from build123d import *

# Parameters (mm, degrees)
ESQUISSE4_R        = 4
ESQUISSE4_R_2      = 3
BOSS_EXTRU_1_DEPTH = 6
ESQUISSE6_R        = 3
ESQUISSE6_R_2      = 1.5
BOSS_EXTRU_2_DEPTH = 1
BOSS_EXTRU_3_DEPTH = 2


with BuildPart() as part:
    # Esquisse4 → Boss.-Extru.1 (new body)
    with BuildSketch(Plane.XY):
        Circle(ESQUISSE4_R)
        Circle(ESQUISSE4_R_2, mode=Mode.SUBTRACT)
    extrude(amount=BOSS_EXTRU_1_DEPTH)

    # Esquisse6 → Boss.-Extru.2 (add)
    with BuildSketch(Plane.XY.offset(6)):
        Circle(ESQUISSE6_R)
        Circle(ESQUISSE6_R_2, mode=Mode.SUBTRACT)
    extrude(amount=-BOSS_EXTRU_2_DEPTH)

    # Esquisse7 → Boss.-Extru.3 (add)
    with BuildSketch(Plane.XY.offset(6)):
        with BuildLine():
            ThreePointArc((3.464101615, 2), (3.863703305, 1.03527618), (4, 0))
            ThreePointArc((4, 0), (3.870082468, -1.011168479), (3.488769153, -1.956652702))
            Line((3.488769153, -1.956652702), (3.505079435, -2))
            Line((3.505079435, -2), (10.76772807, -2))
            Line((10.76772807, -2), (20.627571531, 6.877842929))
            ThreePointArc((20.627571531, 6.877842929), (20.775599969, 9.702393792), (17.951049106, 9.85042223))
            Line((17.951049106, 9.85042223), (9.23227193, 2))
            Line((9.23227193, 2), (3.464101615, 2))
        make_face()
        with BuildLine():
            ThreePointArc((0, 4), (1.03527618, 3.863703305), (2, 3.464101615))
            Line((2, 3.464101615), (2, 9.23227193))
            Line((2, 9.23227193), (9.85042223, 17.951049106))
            ThreePointArc((9.85042223, 17.951049106), (9.702393792, 20.775599969), (6.877842929, 20.627571531))
            Line((6.877842929, 20.627571531), (-2, 10.76772807))
            Line((-2, 10.76772807), (-2, 3.464101615))
            ThreePointArc((-2, 3.464101615), (-1.03527618, 3.863703305), (0, 4))
        make_face()
    extrude(amount=-BOSS_EXTRU_3_DEPTH)


solid = part.part
Input: part model. Units: mm. Frame: model coordinates. A direction names the side the tool comes from. Round coordinates to 2 decimals unless told otherwise and drop trailing zeros. Loops run counter-clockwise (first coordinate to the right, second up) from the corner with the lowest first, then second, coordinate; pieces in that order, holes last. Notation, with made-up numbers: (-31.5, 81) -> (10.5, 81) arc R22 cw to (10.5, 88) -> close; hole circle Ø2 at (50, 6.25). An arc over 180 degrees is marked (long way). Answer as a JSON object with one key per item and string values. Group by question number.
1) Pin query (flat end, axial travel): pin 1 (10 mm diameter, centred on x = 7.5, y = 7.5, fed in from +Z); pin 2 (1.6 mm diameter, centred on x = 6, z = 4.5, fed in from -Y); pin 3 (1.6 mm diameter, centred on y = 8.5, z = 5, fed in from -X); pin 4 (10 mm diameter, centred on x = 15.5, y = 3.5, fed in from -Z). Return the tip coordinate at first contact, or that it passes through.
2) Ray query, L1, parallel to Y at x = 0, z = 3.2; L2, parallel to Z at x = -1.5, y = -2.5; L3, parallel to Z at x = 19.75, y = 6.5. Return the intervals inside material, ascending.
3) Reachability of faces 5 (the cylindrical face through (-3, 0, 2)), 6 (the flat face through (10, 2, 6)), 7 (the flat face through (-2, 7, 5)), 8 (the flat face through (2, 6, 5)), 9 (the flat face through (7, -2, 5)) from +Z, -Z, +X, -X, +Y, -Y: full face, straight path, thin tool, end or side. Return the list, or none.
4) Section query A-A on z = 5.3. Output: boundary loops of the cut face in (x, y), plus the area to 3 significant figures.
5) Section query D-D on x = 8. Output: boundary loops of the cut face in (y, z).
6) Section query B-B on x = 0. Output: boundary loops of the cut face in (y, z).
7) Draft query along X for faces 1 (the flat face through (6, 2, 5)), 2 (the cylindrical face through (9.73, 20.75, 5.01)), 3 (the flat face through (1, 3, 0)), 4 (the flat face through (15.63, 2.38, 5.01)). Return one class per face: +X half, -X half, draft (parallel to the pull), parting line (faces both ways), or undercut.
Reply:
{
 "1": {"pin 1": "passes through", "pin 2": "stops at y = -2", "pin 3": "stops at x = -2", "pin 4": "stops at z = 4"},
 "2": {"L1": "y = -4 to -3, 3 to 4", "L2": "z = 5 to 6", "L3": "z = 4 to 6"},
 "3": {"face 5": "-Z", "face 6": "+Z, +X, -X, +Y, -Y", "face 7": "+Z, -Z, -X, +Y", "face 8": "+Z, -Z", "face 9": "+Z, -Z, +X, -Y"},
 "4": {"outline": "(-2, 3.46) arc R4 ccw (long way) to (3.49, -1.96) -> (3.51, -2) -> (10.77, -2) -> (20.63, 6.88) arc R2 ccw to (17.95, 9.85) -> (9.23, 2) -> (3.46, 2) arc R4 ccw to (2, 3.46) -> (2, 9.23) -> (9.85, 17.95) arc R2 ccw to (6.88, 20.63) -> (-2, 10.77) -> close; hole circle Ø3 at (0, 0)", "area": "205 mm2"},
 "5": {"outline": "(-2, 4) -> (2, 4) -> (2, 6) -> (-2, 6) -> close; (15.9, 4) -> (21.26, 4) -> (21.26, 6) -> (15.9, 6) -> close"},
 "6": {"outline": "(-4, 0) -> (-3, 0) -> (-3, 5) -> (-1.5, 5) -> (-1.5, 6) -> (-4, 6) -> close; (1.5, 5) -> (3, 5) -> (3, 0) -> (4, 0) -> (4, 4) -> (12.99, 4) -> (12.99, 6) -> (1.5, 6) -> close"},
 "7": {"face 1": "undercut", "face 2": "parting line", "face 3": "draft", "face 4": "+X half"}
}
